Geometry: final body of the model. Coordinates: model frame, mm. A direction names the side the tool comes from. Give positions to 0.01 mm unless a question says otherwise; leave off trailing zeros. Write each loop counter-clockwise with the first axis right and the second up, starting at its lowest first coordinate (ties: lowest second). Pieces come first, ordered by that corner, then holes. Notation, with made-up numbers: (-30, -37) -> (-19, -37) arc R6 ccw to (-19, -30) -> close; hole circle Ø4 at (57, -11.5). An arc over 180 degrees is marked (long way). Answer as a JSON object with one key per item and string values.
from build123d import *

# Parameters (mm, degrees)
SKETCH017_R     = 1.9
PAD007_DEPTH    = 8
POCKET010_DEPTH = 3
POCKET011_DEPTH = 4
SKETCH021_W     = 16.2
SKETCH021_H     = 16.2
POCKET012_DEPTH = 1
SKETCH022_R     = 3.2
POCKET013_DEPTH = 3
PAD008_DEPTH    = 5
CHAMFER005_SIZE = 1


with BuildPart() as part:
    # Sketch017 (on Face1 of ShapeBinder001) → Pad007 (new body)
    with BuildSketch(Plane.XY.offset(157)):
        Polygon((0, 38.536997), (-36.650862, 11.908587), (-22.651479, -31.177086), (22.651479, -31.177086), (36.650862, 11.908587), align=None)
        with Locations((-28.478046, 6.171653)):
            Circle(SKETCH017_R, mode=Mode.SUBTRACT)
        with Locations((28.478046, 6.171653)):
            Circle(SKETCH017_R, mode=Mode.SUBTRACT)
        with BuildLine():
            ThreePointArc((-2.291288, 5), (-5.5, 0), (-2.291288, -5))
            Line((-2.291288, -5), (2.291288, -5))
            ThreePointArc((2.291288, -5), (5.5, 0), (2.291288, 5))
            Line((-2.291288, 5), (2.291288, 5))
        make_face(mode=Mode.SUBTRACT)
    extrude(amount=PAD007_DEPTH)

    # Sketch019 (on Face12 of Pad007) → Pocket010 (cut)
    with BuildSketch(Plane(origin=(0, 0, 157), x_dir=(1, 0, 0), z_dir=(0, 0, -1))):
        with BuildLine():
            Line((-27.884018, -1.107353), (-19.018766, 26.177086))
            Line((-19.018766, 26.177086), (19.018766, 26.177086))
            Line((19.018766, 26.177086), (27.884018, -1.107353))
            Line((27.884018, -1.107353), (26.932961, -1.41637))
            ThreePointArc((26.932961, -1.41637), (23.722763, -4.626568), (24.432961, -9.110579))
            Line((26.105291, -11.412344), (24.432961, -9.110579))
            Line((0, -30.378949), (26.105291, -11.412344))
            Line((-26.105291, -11.412344), (0, -30.378949))
            Line((-26.105291, -11.412344), (-24.432961, -9.110579))
            ThreePointArc((-24.432961, -9.110579), (-23.722763, -4.626568), (-26.932961, -1.41637))
            Line((-27.884018, -1.107353), (-26.932961, -1.41637))
        make_face()
    extrude(amount=-POCKET010_DEPTH, mode=Mode.SUBTRACT)

    # CopySketch020 → Pocket011 (cut)
    with BuildSketch(Plane(origin=(0, 0, 157), x_dir=(1, 0, 0), z_dir=(0, 0, -1))):
        Polygon((-31.713466, -10.30433), (0, -33.345512), (31.713466, -10.30433), (32.77148, -11.76056), (0, -35.570434), (-32.77148, -11.76056), align=None)
    extrude(amount=-POCKET011_DEPTH, mode=Mode.SUBTRACT)

    # Sketch021 (on Face31 of Pocket011) → Pocket012 (cut)
    with BuildSketch(Plane(origin=(0, 0, 160), x_dir=(1, 0, 0), z_dir=(0, 0, -1))):
        Rectangle(SKETCH021_W, SKETCH021_H)
    extrude(amount=-POCKET012_DEPTH, mode=Mode.SUBTRACT)

    # Sketch022 (on Face5 of Pocket012) → Pocket013 (cut)
    with BuildSketch(Plane.XY.offset(165)):
        with Locations((-28.478046, 6.171653)):
            Circle(SKETCH022_R)
        with Locations((28.478046, 6.171653)):
            Circle(SKETCH022_R)
    extrude(amount=-POCKET013_DEPTH, mode=Mode.SUBTRACT)

    # Sketch023 (on Face4 of Pocket013) → Pad008 (join)
    with BuildSketch(Plane(origin=(0, 0, 157), x_dir=(1, 0, 0), z_dir=(0, 0, -1))):
        Polygon((-20.563851, 21.421803), (-19.018766, 26.177086), (-14.018766, 26.177086), (-14.018766, 28.577086), (-20.762468, 28.577086), (-22.846387, 22.163444), align=None)
        Polygon((14.018766, 26.177086), (19.018766, 26.177086), (20.563851, 21.421803), (22.846387, 22.163444), (20.762468, 28.577086), (14.018766, 28.577086), align=None)
    extrude(amount=PAD008_DEPTH)

    # Chamfer005
    chamfer005_edges = [part.edges().sort_by_distance(p)[0] for p in [
        (18.325431, 25.222792, 157),
        (-18.325431, 25.222792, 157),
        (29.65117, -9.634249, 157),
        (0, -31.177086, 157),
        (-29.65117, -9.634249, 157),
        (18.325431, 25.222792, 165),
        (29.65117, -9.634249, 165),
        (-18.325431, 25.222792, 165),
        (-29.65117, -9.634249, 165),
        (0, -31.177086, 165),
    ]]
    chamfer(chamfer005_edges, length=CHAMFER005_SIZE)


solid = part.part
Q1. Set-up query: faces 1 (the cylindrical face through (-25.426, 7.133, 163.521)), 2 (the cylindrical face through (5.5, -0.1, 163)), 3 (the flat face through (-25.281, 10.278, 158.479)). Return all of +Z, -Z, +X, -X, +Y, -Y with unobstructed straight access to the full face (end or side cutting, diameter ignored); none if empty.
Values:
{"face 1": "+Z", "face 2": "+Z, -Z", "face 3": "-Z"}
Q2. Cut plane C-C (y = 19). Return the cut outline in (x, z).
Values:
{"outline": "(-26.89, 158) -> (-25.19, 157) -> (-22.81, 157) -> (-22.81, 161) -> (-19.74, 161) -> (-19.74, 157) -> (-15.66, 157) -> (-15.66, 160) -> (15.66, 160) -> (15.66, 157) -> (19.74, 157) -> (19.74, 161) -> (22.81, 161) -> (22.81, 157) -> (25.19, 157) -> (26.89, 158) -> (26.89, 164) -> (25.19, 165) -> (-25.19, 165) -> (-26.89, 164) -> close"}
Q3. Mould query, pull axis Y, two halves, no side actions, for faces 4 (the flat face through (21.689, -21.787, 154.535)), 5 (the flat face through (0, -5, 163)), 6 (the flat face through (21.819, -25.325, 154.535)). Classes: pulls with the +Y half, pulls with the -Y half, needs draft (parallel to the pull), parting line crosses it, or undercut.
Values:
{"face 4": "pulls with the +Y half", "face 5": "undercut", "face 6": "pulls with the -Y half"}
Q4. First-contact query: P1, Ø5, axis at x = -28.48, y = 6.17, coming from the -Z side; P2, Ø1, axis at y = -17.5, z = 157, coming from the +X side; P3, Ø0.5, axis at x = -1.5, z = 160.5, coming from the +Y side; P4, Ø1.5, axis at x = 29, z = 155, coming from the -Y side. Flat tips, straight axial feed; report the tip coordinate or a pass-through.
Values:
{"P1": "z = 157", "P2": "x = 26.59", "P3": "y = 37.63", "P4": "through"}
Q5. Cut plane B-B (y = -3). Return the cut outline in (x, z), and give its area (3 significant figures).
Values:
{"outline": "(-31.81, 158) -> (-30.76, 157) -> (-26.55, 157) -> (-26.55, 160) -> (-8.1, 160) -> (-8.1, 161) -> (-4.61, 161) -> (-4.61, 165) -> (-30.76, 165) -> (-31.81, 164) -> close; (4.61, 161) -> (8.1, 161) -> (8.1, 160) -> (26.55, 160) -> (26.55, 157) -> (30.76, 157) -> (31.81, 158) -> (31.81, 164) -> (30.76, 165) -> (4.61, 165) -> close", "area": "294 mm²"}
Q6. Cut plane D-D (x = -11). Return the cut outline in (y, z).
Values:
{"outline": "(-31.18, 158) -> (-30.18, 157) -> (-26.18, 157) -> (-26.18, 160) -> (22.39, 160) -> (22.39, 157) -> (25.35, 157) -> (25.35, 161) -> (27.58, 161) -> (27.58, 157) -> (29.31, 157) -> (30.55, 158) -> (30.55, 164) -> (29.31, 165) -> (-30.18, 165) -> (-31.18, 164) -> close"}
Q7. Cut plane A-A (z = 154.75). Return the cut outline in (x, y).
Values:
{"outline": "(-22.85, -22.16) -> (-20.76, -28.58) -> (-14.02, -28.58) -> (-14.02, -26.18) -> (-19.02, -26.18) -> (-20.56, -21.42) -> close; (14.02, -28.58) -> (20.76, -28.58) -> (22.85, -22.16) -> (20.56, -21.42) -> (19.02, -26.18) -> (14.02, -26.18) -> close"}
Q8. Material intervals for L1, parallel to Y at x = 10, z = 159.5 (3 decimals); L2, parallel to Y at x = -4.5, z = 160.5; L3, parallel to X at y = 25.5, z = 159.25, sorted ascending. Write a range as from..to.
Values:
{"L1": "-31.177..-26.177, 23.114..26.08, 28.305..31.272", "L2": "-31.18..-8.1, 8.1..30.08, 32.3..35.27", "L3": "-17.94..-13.86, -10.8..-6.72, 6.72..10.8, 13.86..17.94"}
